Build history of the part. All positions in model axes, mm. Give positions to 0.01 mm unless a question says otherwise; leave off trailing zeros. Write each loop counter-clockwise with the first axis right and the second up, starting at its lowest first coordinate (ties: lowest second). Pieces come first, ordered by that corner, then holes. Notation, with made-up numbers: (-40, 67) - (-1, 67) arc R4 ccw to (-1, 71) - close; hole circle Ø5 at (-25.5, -1.75). An arc over 180 degrees is marked (long way). Use one line per item in the form item = value. Start each with the question number.
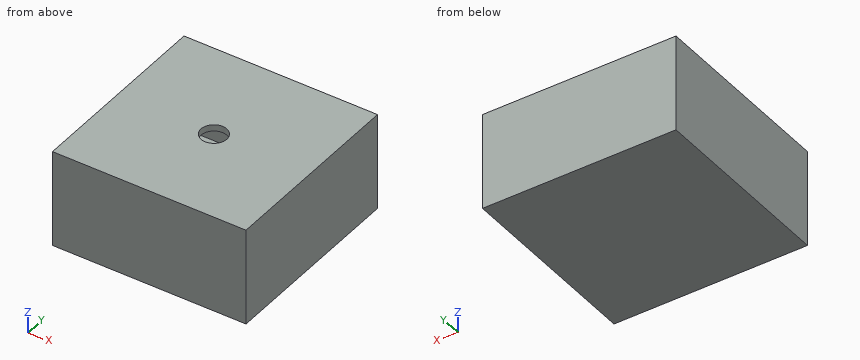
from build123d import *

# Parameters (mm, degrees)
CYLINDER001_R     = 2
CYLINDER001_DEPTH = 3
BOX002_W          = 26
BOX002_H          = 26
BOX002_DEPTH      = 12
BOX001_W          = 30
BOX001_H          = 30
BOX001_DEPTH      = 15


with BuildPart() as cylinder_cut:
    # Cylinder001 → Cylinder001 (new body)
    with BuildSketch(Plane(origin=(15, 14.75, 13), x_dir=(1, 0, 0), z_dir=(0, 0, 1))):
        Circle(CYLINDER001_R)
    extrude(amount=CYLINDER001_DEPTH)


with BuildPart() as box_in:
    # Box002 → Box002 (new body)
    with BuildSketch(Plane(origin=(2, 2, 2), x_dir=(1, 0, 0), z_dir=(0, 0, 1))):
        with Locations((13, 13)):
            Rectangle(BOX002_W, BOX002_H)
    extrude(amount=BOX002_DEPTH)


with BuildPart() as cut001:
    # Box001 → Box001 (new body)
    with BuildSketch(Plane.XY):
        with Locations((15, 15)):
            Rectangle(BOX001_W, BOX001_H)
    extrude(amount=BOX001_DEPTH)

    # Cut: cut Box_in
    add(box_in.part, mode=Mode.SUBTRACT)

    # Cut001: cut Cylinder_cut
    add(cylinder_cut.part, mode=Mode.SUBTRACT)


solid = cut001.part
(1) Cut at B-B, the plane y = 14.75. Give the cut face in (x, z), then the cut area to 3 significant figures.
(2) Cut at D-D, the plane x = 15. Give the cut face in (y, z).
(3) Cut at A-A, the plane z = 5.75. Give the cut face in (x, y).
(4) Pin check, flat tip, straight feed: pin 1 Ø2 at (x, y) = (26, 13) entering from -Z. Stop position of the tip, or through.
(5) Wall check: line 1 (X direction, y = 14.75, z = 14.5); line 2 (Z direction, x = 25.75, y = 10.75); line 3 (X direction, y = 18.5, z = 8.5). Give the ranges that are in metal, low to high. Write a range as from..to.
(6) Cut at C-C, the plane x = 24. Give the cut face in (y, z).
Solution:
q1.outline = (0, 0) - (30, 0) - (30, 15) - (17, 15) - (17, 14) - (28, 14) - (28, 2) - (2, 2) - (2, 14) - (13, 14) - (13, 15) - (0, 15) - close
q1.area = 134 mm2
q2.outline = (0, 0) - (30, 0) - (30, 15) - (16.75, 15) - (16.75, 14) - (28, 14) - (28, 2) - (2, 2) - (2, 14) - (12.75, 14) - (12.75, 15) - (0, 15) - close
q3.outline = (0, 0) - (30, 0) - (30, 30) - (0, 30) - close; hole (2, 2) - (28, 2) - (28, 28) - (2, 28) - close
q4.pin_1 = 0
q5.line_1 = 0..13, 17..30
q5.line_2 = 0..2, 14..15
q5.line_3 = 0..2, 28..30
q6.outline = (0, 0) - (30, 0) - (30, 15) - (0, 15) - close; hole (2, 2) - (28, 2) - (28, 14) - (2, 14) - close
